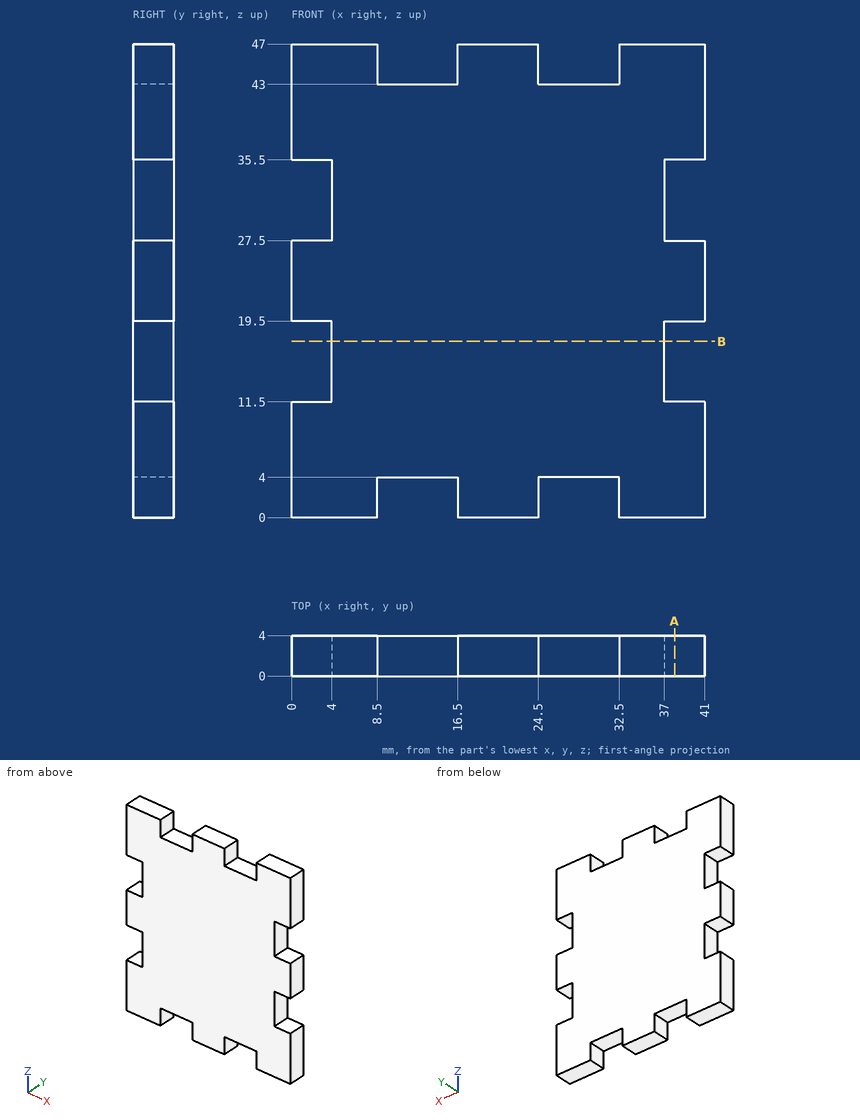
Answer from the drawing. Dimensions are ordinates in mm from the lowest x, y and z of the part. Round coordinates to 2 decimals unless told otherwise and drop trailing zeros. Order: outer loops, then holes, each group sorted by start corner. A loop starts at its lowest first (then second) coordinate and runs counter-clockwise, first axis right, second up. Notation, with made-up numbers: (31.25, -33) -> (50.25, -33) arc R21 ccw to (50.25, -24) -> close; hole circle Ø10 at (3.5, -39). An arc over 180 degrees is marked (long way). Answer as CSV lines item,"result".
Q1. Consider line 1 (Z direction, x = 25.5, y = 2.1); line 2 (X direction, y = 1.8, z = 30). Determine where each line is inside the solid, lowest interval first. Write a range as from..to.
Computed values:
line 1,"z = 4..43"
line 2,"x = 4..37"
Q2. Given pin 1 (1.2 mm diameter, centred on y = 2.5, z = 17, fed in from +X); pin 2 (3 mm diameter, centred on x = 17.5, z = 30, fed in from -Y); pin 3 (2 mm diameter, centred on x = 12, y = 1, fed in from +Z); pin 4 (2 mm diameter, centred on x = 14, y = 2, fed in from -Z), each flat-ended and moving along its own axis, determine where each tip first touches the part or whether it passes through.
Computed values:
pin 1,"stops at x = 37"
pin 2,"stops at y = 0"
pin 3,"stops at z = 43"
pin 4,"stops at z = 4"
Q3. A cutting plane is placed at A-A on x = 38. Determine the outline of the cut face in (y, z).
Computed values:
outline,"(0, 0) -> (4, 0) -> (4, 11.5) -> (0, 11.5) -> close; (0, 19.5) -> (4, 19.5) -> (4, 27.5) -> (0, 27.5) -> close; (0, 35.5) -> (4, 35.5) -> (4, 47) -> (0, 47) -> close"
Q4. A cutting plane is placed at B-B on z = 17.5. Determine the outline of the cut face in (x, y), plus the area to 3 significant figures.
Computed values:
outline,"(4, 0) -> (37, 0) -> (37, 4) -> (4, 4) -> close"
area,"132 mm^2"
